```python
from build123d import *

# Parameters (mm, degrees)
SALIENTE_EXTRUIR1_DEPTH      = 400
SALIENTE_EXTRUIR1_DEPTH_BACK = 0.1
CORTAR_EXTRUIR4_DEPTH        = 10
CROQUIS4_W                   = 0.15
CROQUIS4_H                   = 10
CORTAR_EXTRUIR9_DEPTH        = 0.1


with BuildPart() as part:
    # Croquis1 → Saliente-Extruir1 (new, two sides: drawn at the far end of the back side and taken through both)
    with BuildSketch(Plane(origin=(0, 0, 0), x_dir=(1, 0, 0), z_dir=(0, 1, 0)).offset(-SALIENTE_EXTRUIR1_DEPTH_BACK)):
        with BuildLine():
            Line((34.919955981, -1.488391566), (40.072080634, -1.226803632))
            add(Edge.make_bspline(
                [(40.072080634, -0.488391566), (40.190854748, -0.858541724), (40.072080634, -1.226803632)],
                knots=[0, 0, 0, 1, 1, 1], degree=2))
            Line((40.072080634, -0.488391566), (34.119955981, -0.488391566))
            ThreePointArc((34.119955981, -0.488391566), (33.766402591, -0.634838176), (33.619955981, -0.988391566))
            Line((33.619955981, -0.988391566), (33.619955981, -6.714416127))
            ThreePointArc((33.619955981, -6.714416127), (33.532088016, -6.926548161), (33.319955981, -7.014416127))
            Line((33.319955981, -7.014416127), (6.752124653, -7.014416127))
            ThreePointArc((6.752124653, -7.014416127), (6.539992619, -6.926548161), (6.452124653, -6.714416127))
            Line((6.452124653, -6.714416127), (6.452124653, -0.988391566))
            ThreePointArc((6.452124653, -0.988391566), (6.305678044, -0.634838176), (5.952124653, -0.488391566))
            Line((5.952124653, -0.488391566), (0, -0.488391566))
            add(Edge.make_bspline(
                [(0, -0.488391566), (-0.118774114, -0.858541724), (0, -1.226803632)],
                knots=[0, 0, 0, 1, 1, 1], degree=2))
            Line((0, -1.226803632), (5.152124653, -1.488391566))
            Line((5.152124653, -1.488391566), (5.152124653, -7.314416127))
            ThreePointArc((5.152124653, -7.314416127), (5.357149906, -7.809390874), (5.852124653, -8.014416127))
            Line((5.852124653, -8.014416127), (34.219955981, -8.014416127))
            ThreePointArc((34.219955981, -8.014416127), (34.714930728, -7.809390874), (34.919955981, -7.314416127))
            Line((34.919955981, -7.314416127), (34.919955981, -1.488391566))
        make_face()
    extrude(amount=SALIENTE_EXTRUIR1_DEPTH + SALIENTE_EXTRUIR1_DEPTH_BACK)

    # Croquis2 → Cortar-Extruir4 (cut)
    with BuildSketch(Plane.XY.offset(8.014416127)):
        with BuildLine():
            Line((16.786040317, 38.25), (16.786040317, 46.75))
            ThreePointArc((16.786040317, 46.75), (20.036040317, 50), (23.286040317, 46.75))
            Line((23.286040317, 46.75), (23.286040317, 38.25))
            ThreePointArc((23.286040317, 38.25), (20.036040317, 35), (16.786040317, 38.25))
        make_face()
        with BuildLine():
            Line((16.786040317, 13.25), (16.786040317, 21.75))
            ThreePointArc((16.786040317, 21.75), (20.036040317, 25), (23.286040317, 21.75))
            Line((23.286040317, 21.75), (23.286040317, 13.25))
            ThreePointArc((23.286040317, 13.25), (20.036040317, 10), (16.786040317, 13.25))
        make_face()
        with BuildLine():
            Line((16.786040317, 63.25), (16.786040317, 71.75))
            ThreePointArc((16.786040317, 71.75), (20.036040317, 75), (23.286040317, 71.75))
            Line((23.286040317, 71.75), (23.286040317, 63.25))
            ThreePointArc((23.286040317, 63.25), (20.036040317, 60), (16.786040317, 63.25))
        make_face()
        with BuildLine():
            Line((16.786040317, 88.25), (16.786040317, 96.75))
            ThreePointArc((16.786040317, 96.75), (20.036040317, 100), (23.286040317, 96.75))
            Line((23.286040317, 96.75), (23.286040317, 88.25))
            ThreePointArc((23.286040317, 88.25), (20.036040317, 85), (16.786040317, 88.25))
        make_face()
        with BuildLine():
            Line((16.786040317, 113.25), (16.786040317, 121.75))
            ThreePointArc((16.786040317, 121.75), (20.036040317, 125), (23.286040317, 121.75))
            Line((23.286040317, 121.75), (23.286040317, 113.25))
            ThreePointArc((23.286040317, 113.25), (20.036040317, 110), (16.786040317, 113.25))
        make_face()
        with BuildLine():
            Line((16.786040317, 138.25), (16.786040317, 146.75))
            ThreePointArc((16.786040317, 146.75), (20.036040317, 150), (23.286040317, 146.75))
            Line((23.286040317, 146.75), (23.286040317, 138.25))
            ThreePointArc((23.286040317, 138.25), (20.036040317, 135), (16.786040317, 138.25))
        make_face()
        with BuildLine():
            Line((16.786040317, 163.25), (16.786040317, 171.75))
            ThreePointArc((16.786040317, 171.75), (20.036040317, 175), (23.286040317, 171.75))
            Line((23.286040317, 171.75), (23.286040317, 163.25))
            ThreePointArc((23.286040317, 163.25), (20.036040317, 160), (16.786040317, 163.25))
        make_face()
        with BuildLine():
            Line((16.786040317, 188.25), (16.786040317, 196.75))
            ThreePointArc((16.786040317, 196.75), (20.036040317, 200), (23.286040317, 196.75))
            Line((23.286040317, 196.75), (23.286040317, 188.25))
            ThreePointArc((23.286040317, 188.25), (20.036040317, 185), (16.786040317, 188.25))
        make_face()
        with BuildLine():
            Line((16.786040317, 216.25), (16.786040317, 224.75))
            ThreePointArc((16.786040317, 224.75), (20.036040317, 228), (23.286040317, 224.75))
            Line((23.286040317, 224.75), (23.286040317, 216.25))
            ThreePointArc((23.286040317, 216.25), (20.036040317, 213), (16.786040317, 216.25))
        make_face()
        with BuildLine():
            Line((16.786040317, 244.25), (16.786040317, 252.75))
            ThreePointArc((16.786040317, 252.75), (20.036040317, 256), (23.286040317, 252.75))
            Line((23.286040317, 252.75), (23.286040317, 244.25))
            ThreePointArc((23.286040317, 244.25), (20.036040317, 241), (16.786040317, 244.25))
        make_face()
        with BuildLine():
            Line((16.786040317, 272.25), (16.786040317, 280.75))
            ThreePointArc((16.786040317, 280.75), (20.036040317, 284), (23.286040317, 280.75))
            Line((23.286040317, 280.75), (23.286040317, 272.25))
            ThreePointArc((23.286040317, 272.25), (20.036040317, 269), (16.786040317, 272.25))
        make_face()
        with BuildLine():
            Line((16.786040317, 300.25), (16.786040317, 308.75))
            ThreePointArc((16.786040317, 308.75), (20.036040317, 312), (23.286040317, 308.75))
            Line((23.286040317, 308.75), (23.286040317, 300.25))
            ThreePointArc((23.286040317, 300.25), (20.036040317, 297), (16.786040317, 300.25))
        make_face()
        with BuildLine():
            Line((16.786040317, 328.25), (16.786040317, 336.75))
            ThreePointArc((16.786040317, 336.75), (20.036040317, 340), (23.286040317, 336.75))
            Line((23.286040317, 336.75), (23.286040317, 328.25))
            ThreePointArc((23.286040317, 328.25), (20.036040317, 325), (16.786040317, 328.25))
        make_face()
        with BuildLine():
            Line((16.786040317, 356.25), (16.786040317, 364.75))
            ThreePointArc((16.786040317, 364.75), (20.036040317, 368), (23.286040317, 364.75))
            Line((23.286040317, 364.75), (23.286040317, 356.25))
            ThreePointArc((23.286040317, 356.25), (20.036040317, 353), (16.786040317, 356.25))
        make_face()
        with BuildLine():
            Line((16.786040317, 384.25), (16.786040317, 392.75))
            ThreePointArc((16.786040317, 392.75), (20.036040317, 396), (23.286040317, 392.75))
            Line((23.286040317, 392.75), (23.286040317, 384.25))
            ThreePointArc((23.286040317, 384.25), (20.036040317, 381), (16.786040317, 384.25))
        make_face()
    extrude(amount=-CORTAR_EXTRUIR4_DEPTH, mode=Mode.SUBTRACT)

    # Croquis4 → Cortar-Extruir9 (cut)
    with BuildSketch(Plane(origin=(0, 0, 7.014416127), x_dir=(-1, 0, 0), z_dir=(0, 0, -1))):
        with Locations((-20.036040317, 29.95)):
            Rectangle(CROQUIS4_W, CROQUIS4_H)
        with Locations((-20.036040317, 4.95)):
            Rectangle(CROQUIS4_W, CROQUIS4_H)
        with Locations((-20.036040317, 54.95)):
            Rectangle(CROQUIS4_W, CROQUIS4_H)
        with Locations((-20.036040317, 79.95)):
            Rectangle(CROQUIS4_W, CROQUIS4_H)
        with Locations((-20.036040317, 104.95)):
            Rectangle(CROQUIS4_W, CROQUIS4_H)
        with Locations((-20.036040317, 129.95)):
            Rectangle(CROQUIS4_W, CROQUIS4_H)
        with Locations((-20.036040317, 154.95)):
            Rectangle(CROQUIS4_W, CROQUIS4_H)
        with Locations((-20.036040317, 179.95)):
            Rectangle(CROQUIS4_W, CROQUIS4_H)
    extrude(amount=-CORTAR_EXTRUIR9_DEPTH, mode=Mode.SUBTRACT)


solid = part.part
```
Design review of the part built by this model. Coordinates are the model's own, in mm. Round coordinates to 2 decimals unless told otherwise and drop trailing zeros. Write each loop counter-clockwise with the first axis right and the second up, starting at its lowest first coordinate (ties: lowest second). Pieces come first, ordered by that corner, then holes. Notation, with made-up numbers: (-6, 64.5) -> (24, 64.5) arc R17 ccw to (24, 81.5) -> close; hole circle Ø8 at (78, 7.25). An arc over 180 degrees is marked (long way). Answer in a Markdown table with one row per item.
Q1. Take a section at A-A, the plane z = 5.5. State the section outline as (x, y) points, then the cut area to 3 significant figures.
The answers:
| item | result |
|---|---|
| outline | (5.15, -0.1) -> (6.45, -0.1) -> (6.45, 400) -> (5.15, 400) -> close; (33.62, -0.1) -> (34.92, -0.1) -> (34.92, 400) -> (33.62, 400) -> close |
| area | 1,040 mm² |
Q2. Take a section at B-B, the plane x = 30. State the section outline as (y, z) points.
The answers:
| item | result |
|---|---|
| outline | (-0.1, 7.01) -> (400, 7.01) -> (400, 8.01) -> (-0.1, 8.01) -> close |
Q3. Clearance check with flat-ended pins moving along their axes: pin 1 Ø2 at (y, z) = (220, 7) entering from -X; pin 2 Ø0.8 at (y, z) = (116, 7.5) entering from +X. State where each tip first meets the part, or that it passes through.
The answers:
| item | result |
|---|---|
| pin 1 | x = 5.15 |
| pin 2 | x = 34.92 |
Q4. Draft analysis for pull direction X (two halves, no side actions). For faces 1 (the face through (22.9, 400, 7.6)), 2 (the face through (26, 197, 7.014)), state which applies: +X half, -X half, draft (parallel to the pull), parting line (faces both ways), or undercut.
The answers:
| item | result |
|---|---|
| face 1 | draft |
| face 2 | undercut |
Q5. To check wall thickness, follow L1, parallel to X at y = 32, z = 5.75; L2, parallel to Z at x = 6, y = 248; L3, parallel to Z at x = 15, y = 367. State the ranges of each line that lie inside material, in increasing order. Write a range as [from, to].
The answers:
| item | result |
|---|---|
| L1 | [5.15, 6.45], [33.62, 34.92] |
| L2 | [0.49, 8.01] |
| L3 | [7.01, 8.01] |
